```python
from build123d import *

# Parameters (mm, degrees)
SKETCH2_W           = 20
SKETCH2_H           = 150
BOSS_EXTRUDE2_DEPTH = 125
SKETCH3_R           = 5
BOSS_EXTRUDE3_DEPTH = 50


with BuildPart() as part:
    # Sketch2 → Boss-Extrude2 (new, symmetric)
    with BuildSketch(Plane(origin=(0, 0, 0), x_dir=(0, 0, -1), z_dir=(1, 0, 0))):
        with Locations((0, 75)):
            Rectangle(SKETCH2_W, SKETCH2_H)
    extrude(amount=BOSS_EXTRUDE2_DEPTH, both=True)

    # Sketch3 → Boss-Extrude3 (add)
    with BuildSketch(Plane.XZ):
        with Locations(Location((-62.5, 0, 0), (0, 0, 90))):
            Circle(SKETCH3_R)
    boss_extrude3 = extrude(amount=BOSS_EXTRUDE3_DEPTH)

    # Mirror1: Boss-Extrude3 across plane
    add(boss_extrude3.mirror(Plane(origin=(0, 0, 0), x_dir=(0, 0, 1), z_dir=(1, 0, 0))))


solid = part.part
```
Verification items for the finished model (mm, model axes). A direction names the side the tool comes from. Give positions to 0.01 mm unless a question says otherwise; leave off trailing zeros. Order: outer loops, then holes, each group sorted by start corner. A loop starts at its lowest first (then second) coordinate and runs counter-clockwise, first axis right, second up. Notation, with made-up numbers: M -17,-0.75 L 28,-0.75 A14 cw 28,23.25 Z; hole C 52.5,81 d9. An arc over 180 degrees is marked long. Answer in a Markdown table with one row per item. Add a question column.
Item 1: Section check B-B, the plane x = 62.5. Enter the section's corners in (y, z), and give its area (3 significant figures).
Item 2: Mould release check, pull along X, two halves, no side actions. Record for faces 1 (the flat face through (125, 76, 0)), 2 (the flat face through (63, -50, 0)), 3 (the cylindrical face through (66.716, -24.65, 2.688)): released by +X, released by -X, zero draft, split by the parting line, or undercut.
Item 3: Section check C-C, the plane x = -28. Enter the section's corners in (y, z).
Item 4: Scan lines: probe 1 along Y at (x, z) = (44.5, -7.75); probe 2 along X at (y, z) = (-37.5, -1). Record each from-to range of solid material in increasing order. Write a range as from..to.
Item 5: Gauge pin test, flat end, axial feed: pin 1 (4 mm diameter, centred on x = -90, z = 8, fed in from -Y). Record the tip position at first contact, or that the pin passes through.
Item 6: Tool access check on faces 4 (the flat face through (-63, -50, 0)), 5 (the cylindrical face through (-66.716, -24.65, 2.688)). Record the directions out of +Z, -Z, +X, -X, +Y, -Y that give a thin tool (end or side, any length) a straight path to the whole face; none if there is none.
Item 7: Section check A-A, the plane y = -29. Enter the section's corners in (x, z), and give its area (3 significant figures).
Filled sheet:
| question | item | result |
|---|---|---|
| 1 | outline | M -50,-5 L 0,-5 L 0,-10 L 150,-10 L 150,10 L 0,10 L 0,5 L -50,5 Z |
| 1 | area | 3,500 mm^2 |
| 2 | face 1 | released by +X |
| 2 | face 2 | zero draft |
| 2 | face 3 | undercut |
| 3 | outline | M 0,-10 L 150,-10 L 150,10 L 0,10 Z |
| 4 | probe 1 | y = 0..150 |
| 4 | probe 2 | x = -67.4..-57.6, 57.6..67.4 |
| 5 | pin 1 | stops at y = 0 |
| 6 | face 4 | +Z, -Z, +X, -X, -Y |
| 6 | face 5 | -Y |
| 7 | outline | C -62.5,0 d10; C 62.5,0 d10 |
| 7 | area | 157 mm^2 |
